Check sheet for the drawn part. Datum: minimum x, y, z corner. Units: mm. Round coordinates to 2 decimals unless told otherwise and drop trailing zeros. Order: outer loops, then holes, each group sorted by start corner. A loop starts at its lowest first (then second) coordinate and runs counter-clockwise, first axis right, second up. Notation, with made-up numbers: (-11, -25.5) -> (5, -25.5) arc R16 ccw to (5, -6.5) -> close; hole circle Ø6 at (74, -23). An arc over 180 degrees is marked (long way). Use CSV: the item, a comma, the result in double quotes.
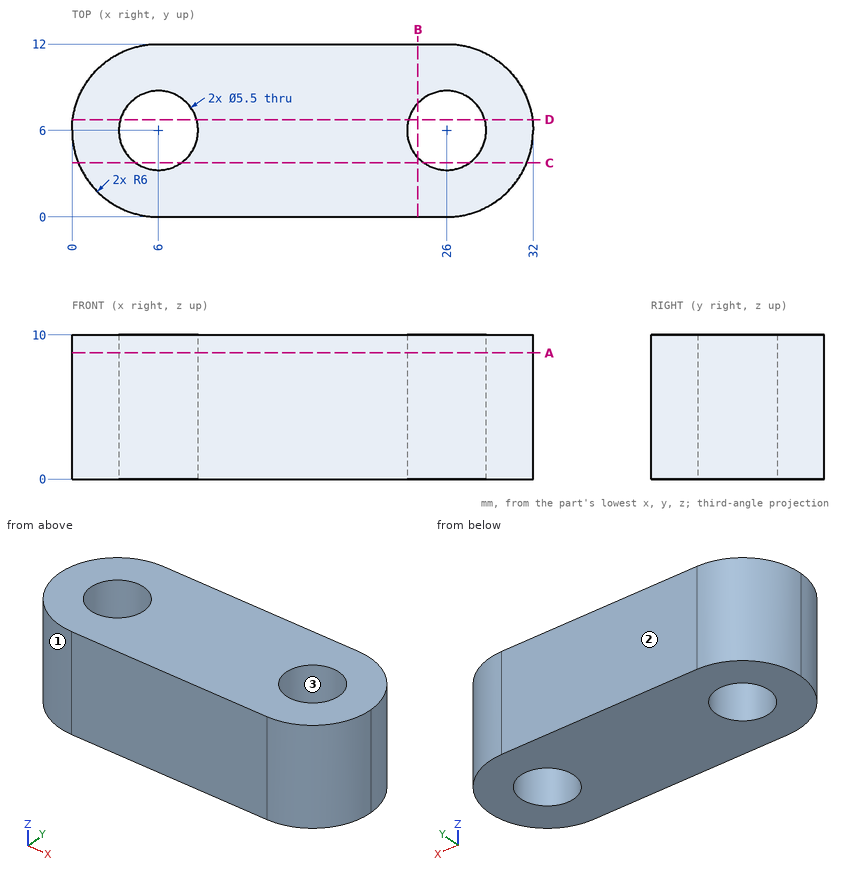
Q1. Sectioned sample at D-D, the plane y = 6.75. Enter the section's corners in (x, z), then the cut area to 3 significant figures.
Result sheet:
outline,"(0.05, 0) -> (3.35, 0) -> (3.35, 10) -> (0.05, 10) -> close; (8.65, 0) -> (23.35, 0) -> (23.35, 10) -> (8.65, 10) -> close; (28.65, 0) -> (31.95, 0) -> (31.95, 10) -> (28.65, 10) -> close"
area,"213 mm^2"
Q2. Mould release check, pull along X, two halves, no side actions. Record for the marked faces 1, 2 and 3: pulls with the +X half, pulls with the -X half, needs draft (parallel to the pull), parting line crosses it, or undercut.
Result sheet:
face 1,"pulls with the -X half"
face 2,"needs draft"
face 3,"undercut"
Q3. Go/stop test with flat-tipped pins: pin 1 (2 mm diameter, centred on y = 1.5, z = 6, fed in from -X); pin 2 (4.5 mm diameter, centred on x = 6, y = 6, fed in from -Z). Record where each tip stops, or that it passes through.
Result sheet:
pin 1,"stops at x = 1.13"
pin 2,"passes through"
Q4. Scan lines: L1, parallel to Y at x = 26, z = 5; L2, parallel to X at y = 3.5, z = 9.75; L3, parallel to X at y = 6.75, z = 4.75. Record each from-to range of solid material in increasing order.
Result sheet:
L1,"y = 0 to 3.25, 8.75 to 12"
L2,"x = 0.55 to 4.85, 7.15 to 24.85, 27.15 to 31.45"
L3,"x = 0.05 to 3.35, 8.65 to 23.35, 28.65 to 31.95"
Q5. Sectioned sample at B-B, the plane x = 24. Enter the section's corners in (y, z).
Result sheet:
outline,"(0, 0) -> (4.11, 0) -> (4.11, 10) -> (0, 10) -> close; (7.89, 0) -> (12, 0) -> (12, 10) -> (7.89, 10) -> close"
Q6. Sectioned sample at A-A, the plane z = 8.75. State how many separate pieces and enclosed holes the cut face has, then the cut area to 3 significant figures.
Result sheet:
separate pieces,"1"
enclosed holes,"2"
area,"306 mm^2"
Q7. Sectioned sample at C-C, the plane y = 3.75. Enter the section's corners in (x, z), then the cut area to 3 significant figures.
Result sheet:
outline,"(0.44, 0) -> (4.42, 0) -> (4.42, 10) -> (0.44, 10) -> close; (7.58, 0) -> (24.42, 0) -> (24.42, 10) -> (7.58, 10) -> close; (27.58, 0) -> (31.56, 0) -> (31.56, 10) -> (27.58, 10) -> close"
area,"248 mm^2"
